Part model, mm, in its own coordinate system. A direction names the side the tool comes from. Give positions to 0.01 mm unless a question says otherwise; leave off trailing zeros. Order: outer loops, then holes, each group sorted by start corner. A loop starts at its lowest first (then second) coordinate and runs counter-clockwise, first axis right, second up. Notation, with made-up numbers: (-1.75, -24) - (51.25, -24) arc R23 ccw to (51.25, 6) - close; hole circle Ø7 at (20, -17.5). An arc over 180 degrees is marked (long way). One line per item, written item: value.
```python
from build123d import *

# Parameters (mm, degrees)
F1_DEPTH = 40
F2_SIZE  = 25
F3_W     = 20
F3_H     = 20
F4_DEPTH = 30
F5_W     = 15
F5_H     = 5
F6_DEPTH = 150
F7_R     = 35
F8_DEPTH = 2


with BuildPart() as f1:
    # F0 (on Top) → F1 (new body)
    with BuildSketch(Plane.XY):
        Polygon((-77.942286, 45), (0, -90), (77.942286, 45), align=None)
    extrude(amount=F1_DEPTH)

    # F2
    f2_edges = [f1.edges().sort_by_distance(p)[0] for p in [
        (0, -90, 20),
        (77.942286, 45, 20),
        (-77.942286, 45, 20),
    ]]
    chamfer(f2_edges, length=F2_SIZE)

    # F3 (on face) → F4 (cut)
    with BuildSketch(Plane.XY.offset(40)):
        with Locations((0, -53.349365)):
            Rectangle(F3_W, F3_H)
        Polygon((-59.862159, 23.014428), (-42.541651, 13.014428), (-32.541651, 30.334936), (-49.862159, 40.334936), align=None)
        Polygon((49.862159, 40.334936), (32.541651, 30.334936), (42.541651, 13.014428), (59.862159, 23.014428), align=None)
    extrude(amount=-F4_DEPTH, mode=Mode.SUBTRACT)

    # F5 (on face) → F6 (join)
    with BuildSketch(Plane.XY.offset(40)):
        with Locations((-17.5, 40)):
            Rectangle(F5_W, F5_H)
        with Locations((17.5, 40)):
            Rectangle(F5_W, F5_H)
        Polygon((41.80608, -12.589746), (49.30608, 0.400635), (44.975953, 2.900635), (37.475953, -10.089746), align=None)
        Polygon((31.80608, -29.910254), (27.475953, -27.410254), (19.975953, -40.400635), (24.30608, -42.900635), align=None)
        Polygon((-31.80608, -29.910254), (-24.30608, -42.900635), (-19.975953, -40.400635), (-27.475953, -27.410254), align=None)
        Polygon((-41.80608, -12.589746), (-37.475953, -10.089746), (-44.975953, 2.900635), (-49.30608, 0.400635), align=None)
    extrude(amount=F6_DEPTH)

    # F7 (on face) → F8 (join)
    with BuildSketch(Plane.XY.offset(40)):
        Circle(F7_R)
    extrude(amount=F8_DEPTH)


solid = f1.part
```
1) Mould opens along Y. For faces 1 (the flat face through (-1, 2, 0)), 2 (the flat face through (-23.67, -34, 113.95)), 3 (the flat face through (-41.081, 35.265, 25.21)), 4 (the flat face through (-39.34, -21.86, 19.72)) say: released by +Y, released by -Y, zero draft, split by the parting line, or undercut.
Outcome:
face 1: zero draft
face 2: undercut
face 3: undercut
face 4: released by -Y
2) Pin check, flat tips, straight feed: pin 1 (3 mm diameter, centred on x = 28.5, y = 6.5, fed in from +Z); pin 2 (4 mm diameter, centred on y = -2.5, z = 60, fed in from -X); pin 3 (10 mm diameter, centred on x = 4.5, y = -57, fed in from +Z). Stop position of each tip, or through.
Outcome:
pin 1: stops at z = 42
pin 2: stops at x = -48.79
pin 3: stops at z = 10
3) Cut at A-A, the plane z = 90. Give the cut face in (x, y).
Outcome:
outline: (-49.31, 0.4) - (-41.81, -12.59) - (-37.48, -10.09) - (-44.98, 2.9) - close; (-31.81, -29.91) - (-24.31, -42.9) - (-19.98, -40.4) - (-27.48, -27.41) - close; (-25, 37.5) - (-10, 37.5) - (-10, 42.5) - (-25, 42.5) - close; (10, 37.5) - (25, 37.5) - (25, 42.5) - (10, 42.5) - close; (19.98, -40.4) - (24.31, -42.9) - (31.81, -29.91) - (27.48, -27.41) - close; (37.48, -10.09) - (41.81, -12.59) - (49.31, 0.4) - (44.98, 2.9) - close
4) Drill centre lines: line 1 along X through (y, z) = (40, 121); line 2 along Z through (x, y) = (-35.5, -24.5); line 3 along Z through (x, y) = (-4.5, -34). Where is each one in solid material? Low to high. Write a range as from..to.
Outcome:
line 1: x = -25..-10, 10..25
line 2: z = 0..40
line 3: z = 0..42
5) Cut at B-B, the plane x = 0. Give the cut face in (y, z), then the cut area to 3 significant figures.
Outcome:
outline: (-68.35, 0) - (45, 0) - (45, 40) - (35, 40) - (35, 42) - (-35, 42) - (-35, 40) - (-43.35, 40) - (-43.35, 10) - (-63.35, 10) - (-63.35, 40) - (-68.35, 40) - close
area: 4,070 mm^2
6) Which spindle directions (+Z, -Z, +X, -X, +Y, -Y) get a long thin tool onto all of the face, cutting with end or side? Do faces 5 (the flat face through (-47.11, 1.67, 113.95)), 6 (the flat face through (17, 37.5, 114)), 7 (the flat face through (54.932, 31.553, 25.21)), 8 (the flat face through (-45.61, -6, 113.95)). Say none if no direction does.
Outcome:
face 5: +Z, -X, +Y
face 6: +Z, +X, -X
face 7: +Z
face 8: +Z, -X, -Y
